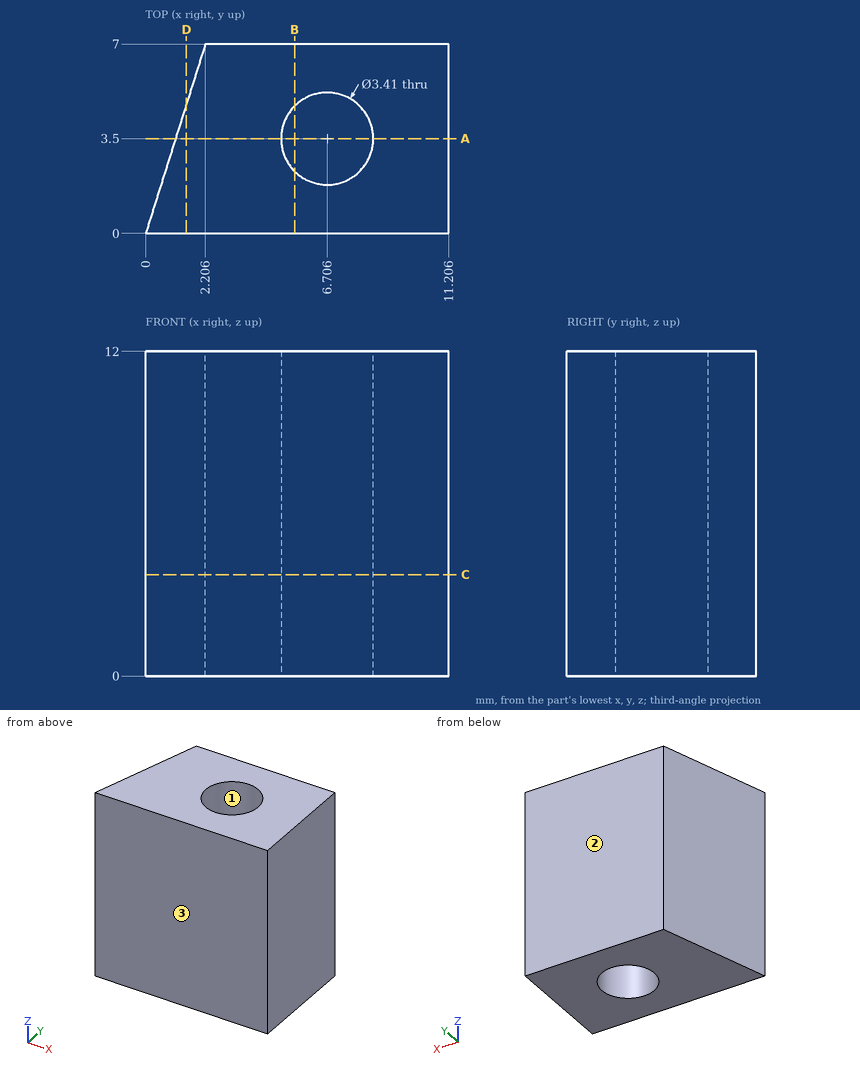
Study the drawing (mm; zero at the part's minimum x, y, z) and answer. Coordinates: 2 decimals unless noted, no trailing zeros. Write each loop counter-clockwise with the first axis right and the second up, starting at its lowest first coordinate (ties: lowest second). Pieces come first, ordered by that corner, then holes. Notation, with made-up numbers: (4.25, 37.5) - (50.25, 37.5) arc R25 ccw to (50.25, 51.5) - close; hole circle Ø4 at (-9.5, 71). An arc over 180 degrees is marked (long way). Answer as a JSON object with one key per item and string values. Group by question number.
1. This flat-tipped pin is pushed along its axis until it touches: P1, Ø5, axis at x = 9, z = 6.5, coming from the -Y side. Where does it stop, or does it pass through?
2. The mould has two halves that part along Y. Classify the marked faces 1, 2 and 3: +Y half, -Y half, draft (parallel to the pull), parting line (faces both ways), or undercut.
3. A cutting plane is placed at A-A (y = 3.5). Determine the outline of the cut face in (x, z).
4. A cutting plane is placed at C-C (z = 3.75). Determine the outline of the cut face in (x, y) (1 decimal), plus the area to 3 significant figures.
5. A cutting plane is placed at B-B (x = 5.5). Determine the outline of the cut face in (y, z) (1 decimal).
6. A cutting plane is placed at D-D (x = 1.5). Determine the outline of the cut face in (y, z), plus the area to 3 significant figures.
7. Consider L1, parallel to X at y = 5, z = 10 (1 decimal); L2, parallel to Y at x = 6.5, z = 2.75; L3, parallel to Y at x = 7.25, z = 10.75 (1 decimal). Determine where each line is inside the solid, lowest interval first. Write a range as [from, to].
Worked out:
{
 "1": {"P1": "stops at y = 0"},
 "2": {"face 1": "undercut", "face 2": "+Y half", "face 3": "-Y half"},
 "3": {"outline": "(1.1, 0) - (5, 0) - (5, 12) - (1.1, 12) - close; (8.41, 0) - (11.21, 0) - (11.21, 12) - (8.41, 12) - close"},
 "4": {"outline": "(0, 0) - (11.2, 0) - (11.2, 7) - (2.2, 7) - close; hole circle Ø3.4 at (6.7, 3.5)", "area": "61.6 mm²"},
 "5": {"outline": "(0, 0) - (2.3, 0) - (2.3, 12) - (0, 12) - close; (4.7, 0) - (7, 0) - (7, 12) - (4.7, 12) - close"},
 "6": {"outline": "(0, 0) - (4.76, 0) - (4.76, 12) - (0, 12) - close", "area": "57.1 mm²"},
 "7": {"L1": "x = [1.6, 5.9], [7.5, 11.2]", "L2": "y = [0, 1.81], [5.19, 7]", "L3": "y = [0, 1.9], [5.1, 7]"}
}
